Work out the finished part from the listing and answer in its coordinate system (mm). A direction names the side the tool comes from. Coordinates: 2 decimals unless noted, no trailing zeros. Write each loop counter-clockwise with the first axis right and the second up, starting at its lowest first coordinate (ties: lowest second). Pieces come first, ordered by that corner, then holes. Notation, with made-up numbers: M -19,57.25 L 7,57.25 A31 ccw 7,96.25 Z; hole C 7.5,-11 d8. An arc over 180 degrees is marked long. Use CSV: the item, a comma, the result in double quotes.
Autodesk Fusion 360 part; units mm, degrees
sketch "Sketch1" plane through (0, 0, 0) normal (0, 1, 0) x (1, 0, 0)
  line L0 (47, 0) -> (47, -22)
  line L1 (47, -22) -> (45, -22)
  line L2 (45, -22) -> (45, -12)
  line L3 (45, -12) -> (35, -12)
  line L4 (35, -12) -> (35, -10)
  line L5 (35, -10) -> (45, -10)
  line L6 (45, -10) -> (45, 0)
  line L7 (45, 0) -> (47, 0)
  dimension "d1" = 45
  dimension "d2" = 35
  dimension "d3" = 2
  dimension "d4" = 2
  dimension "d5" = 10
revolve "Revolve1" add sketch "Sketch1" angle 360 about axis through (0, 0, 1.75) along (0, 0, 1)
Item 1: The part is cut by section A-A (x = 0). Write down the section's boundary in (y, z), then the cut area to 3 significant figures.
Answer:
outline,"M -47,0 L -45,0 L -45,10 L -35,10 L -35,12 L -45,12 L -45,22 L -47,22 Z; M 35,10 L 45,10 L 45,0 L 47,0 L 47,22 L 45,22 L 45,12 L 35,12 Z"
area,"128 mm2"
Item 2: A tool of negligible diameter and unlimited length cuts with its end or side. For faces 4 (the face through (-28, 21, 11)), 5 (the face through (23.1, -26.5, 12)), 6 (the face through (23.1, -26.5, 10)), from which of +Z, -Z, +X, -X, +Y, -Y can it reach the whole face along a straight path? Write none if from no direction.
Answer:
face 4,"+Z, -Z"
face 5,"+Z"
face 6,"-Z"
Item 3: Given pin 1 (2 mm diameter, centred on y = -10, z = 3, fed in from -X); pin 2 (2 mm diameter, centred on x = 27, z = 14, fed in from -Y); pin 3 (1 mm diameter, centred on x = 30.5, y = -28, fed in from -Z), each flat-ended and moving along its own axis, determine where each tip first touches the part or whether it passes through.
Answer:
pin 1,"stops at x = -46.13"
pin 2,"stops at y = -39.15"
pin 3,"stops at z = 10"
Item 4: The part is cut by section C-C (z = 3.75). Write down the section's boundary in (x, y).
Answer:
outline,"C 0,0 d94; hole C 0,0 d90"
Item 5: For a pull along Y with two mould halves and no side action, classify faces 1 (the face through (20.765, 39.923, 4.93)), 2 (the face through (44.83, 14.12, 11.15)), 3 (the face through (45.04, -3.26, 22)) as released by +Y, released by -Y, zero draft, split by the parting line, or undercut.
Answer:
face 1,"undercut"
face 2,"split by the parting line"
face 3,"zero draft"
Item 6: Consider probe 1 along Y at (x, z) = (0, 18); probe 2 along Y at (x, z) = (0, 11.15); probe 3 along X at (y, z) = (20.5, 3.75). Determine where each line is inside the solid, lowest interval first.
Answer:
probe 1,"y = -47 to -45, 45 to 47"
probe 2,"y = -47 to -35, 35 to 47"
probe 3,"x = -42.29 to -40.06, 40.06 to 42.29"
Item 7: The part is cut by section D-D (y = -37.5). Write down the section's boundary in (x, z), then the cut area to 3 significant figures.
Answer:
outline,"M -28.33,0 L -24.87,0 L -24.87,10 L 24.87,10 L 24.87,0 L 28.33,0 L 28.33,22 L 24.87,22 L 24.87,12 L -24.87,12 L -24.87,22 L -28.33,22 Z"
area,"252 mm2"
